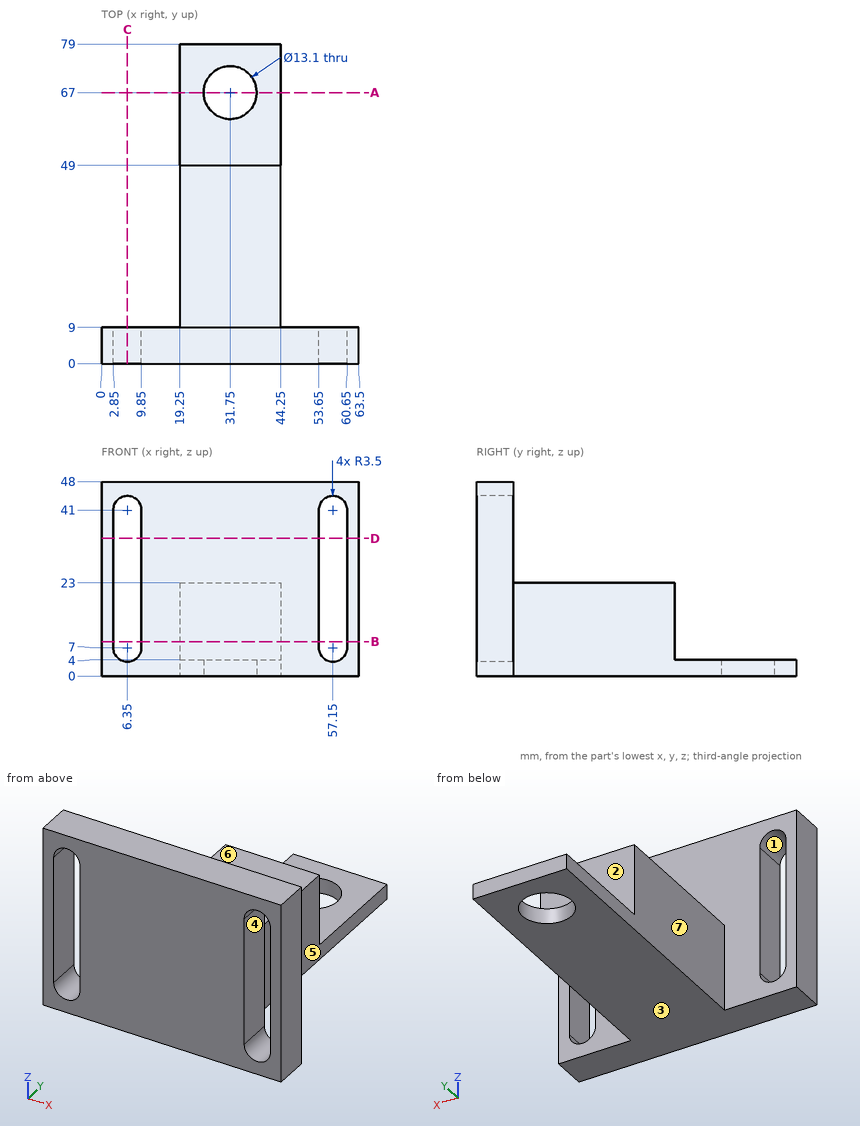
Can you work these out from the drawing? Everything is in mm from the part's minimum corner. A direction names the side the tool comes from. Coordinates: 2 decimals unless noted, no trailing zeros. Loops run counter-clockwise (first coordinate to the right, second up) from the corner with the lowest first, then second, coordinate; pieces in that order, holes last.
1) Imagine slicing it at B-B (z = 8.5). List the corners of the cut face in (x, y) for me, and give its area (3 significant figures).
Reported:
outline: (0, 0) - (2.85, 0) - (2.85, 9) - (0, 9) - close; (9.85, 0) - (53.65, 0) - (53.65, 9) - (44.25, 9) - (44.25, 49) - (19.25, 49) - (19.25, 9) - (9.85, 9) - close; (60.65, 0) - (63.5, 0) - (63.5, 9) - (60.65, 9) - close
area: 1,450 mm2
2) Imagine slicing it at A-A (y = 67). List the corners of the cut face in (x, z) for me.
Reported:
outline: (19.25, 0) - (25.2, 0) - (25.2, 4) - (19.25, 4) - close; (38.3, 0) - (44.25, 0) - (44.25, 4) - (38.3, 4) - close
3) Please list where these lines run through material, in increasing order: line 1 along X through (y, z) = (6.5, 32); line 2 along Y through (x, z) = (31.75, 1.95); line 3 along X through (y, z) = (67, 2.7).
Reported:
line 1: x = 0 to 2.85, 9.85 to 53.65, 60.65 to 63.5
line 2: y = 0 to 60.45, 73.55 to 79
line 3: x = 19.25 to 25.2, 38.3 to 44.25
4) Which directions (+Z, -Z, +X, -X, +Y, -Y) give clear straight access to the entire face, cutting with the end or side of a thin tool? Please do the marked faces 4, 5, 6 and 7.
Reported:
face 4: +Y, -Y
face 5: +Z, -Z, +X, +Y
face 6: +Z, +X, -X, +Y
face 7: +Z, -Z, -X, +Y
5) Will these pins go through, and if not, where does the flat tip stop? pin 1 Ø11.5 at (y, z) = (41.5, 6) entering from +X; pin 2 Ø20 at (x, y) = (30.5, 29) entering from +Z; pin 3 Ø10 at (x, z) = (45, 11.5) entering from +Y.
Reported:
pin 1: stops at x = 44.25
pin 2: stops at z = 23
pin 3: stops at y = 49
6) Thinking about a two-plate mould opening in Z: for the marked faces 1, 2 and 3, which applies, released by +Z, released by -Z, zero draft, split by the parting line, or undercut?
Reported:
face 1: undercut
face 2: zero draft
face 3: released by -Z
7) Imagine slicing it at D-D (z = 34). List the corners of the cut face in (x, y) for me, and give its area (4 significant figures).
Reported:
outline: (0, 0) - (2.85, 0) - (2.85, 9) - (0, 9) - close; (9.85, 0) - (53.65, 0) - (53.65, 9) - (9.85, 9) - close; (60.65, 0) - (63.5, 0) - (63.5, 9) - (60.65, 9) - close
area: 445.5 mm2
8) Imagine slicing it at C-C (x = 6.35). List the corners of the cut face in (y, z) for me, and give its area (3 significant figures).
Reported:
outline: (0, 0) - (9, 0) - (9, 3.5) - (0, 3.5) - close; (0, 44.5) - (9, 44.5) - (9, 48) - (0, 48) - close
area: 63.0 mm2
